Can you work these out from the drawing? Everything is in mm from the part's minimum corner. Give positions to 0.01 mm unless a question says otherwise; leave off trailing zeros. Write each loop counter-clockwise with the first axis right and the second up, starting at its lowest first coordinate (ties: lowest second). Pieces come first, ordered by that corner, then holes. Notation, with made-up numbers: (3, 72) - (14, 72) arc R21 ccw to (14, 78) - close; hole circle Ø7 at (20, 65). An arc over 180 degrees is marked (long way). Return JSON: item names as keys, results as strings. Group by question number.
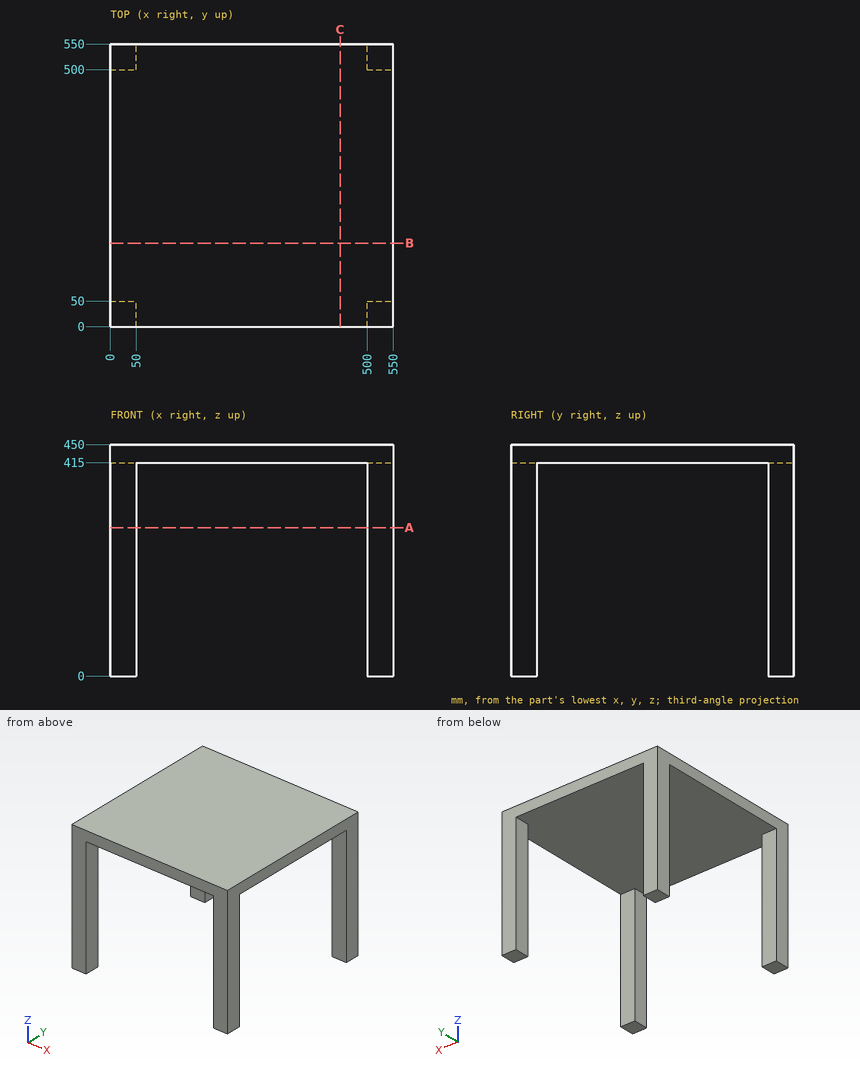
1) Imagine slicing it at B-B, the plane y = 162.5. Write out the boundary of the cut face in (x, z), and give its area (4 significant figures).
2) I need wall thicknesses on line 1 along X through (y, z) = (520.5, 346.5); line 2 along Z through (x, y) = (234, 285). Which ranges of each line are inside material? Lowest first, please.
3) Will this pin go through, and if not, where does the flat tip stop? pin 1 Ø4 at (x, y) = (408, 345.5) entering from -Z.
4) Imagine slicing it at A-A, the plane z = 288.5. Write out the boundary of the cut face in (x, y), and give its area (3 significant figures).
Resolved:
{
 "1": {"outline": "(0, 415) - (550, 415) - (550, 450) - (0, 450) - close", "area": "19,250 mm^2"},
 "2": {"line 1": "0 to 50, 500 to 550", "line 2": "415 to 450"},
 "3": {"pin 1": "z = 415"},
 "4": {"outline": "(0, 0) - (50, 0) - (50, 50) - (0, 50) - close; (0, 500) - (50, 500) - (50, 550) - (0, 550) - close; (500, 0) - (550, 0) - (550, 50) - (500, 50) - close; (500, 500) - (550, 500) - (550, 550) - (500, 550) - close", "area": "10,000 mm^2"}
}
